Read the model definition and answer for the solid it produces. Units are mm, in the model's axes. Face numbers are marked on the shaded views. Coordinates: 2 decimals unless noted, no trailing zeros. Write each loop counter-clockwise with the first axis right and the second up, starting at its lowest first coordinate (ties: lowest second). Pieces come first, ordered by that corner, then holes. Notation, with made-up numbers: (4.5, -39.5) -> (56.5, -39.5) arc R11 ccw to (56.5, -31.5) -> close; hole circle Ø1 at (-16.5, 41.25). An arc over 180 degrees is marked (long way). Return JSON: item names as keys, results as strings.
from build123d import *

# Parameters (mm, degrees)
SKETCH1_R           = 6.1
SKETCH1_R_2         = 1.5
BOSS_EXTRUDE1_DEPTH = 2.3
SKETCH2_R           = 4.4
SKETCH2_R_2         = 3
BOSS_EXTRUDE2_DEPTH = 3.2
SKETCH3_R           = 0.75
BOSS_EXTRUDE3_DEPTH = 2.3
CIRPATTERN1_COUNT   = 6


with BuildPart() as part:
    # Sketch1 → Boss-Extrude1 (new body)
    with BuildSketch(Plane(origin=(0, 0, 0), x_dir=(1, 0, 0), z_dir=(0, 1, 0))):
        Circle(SKETCH1_R)
        Circle(SKETCH1_R_2, mode=Mode.SUBTRACT)
    extrude(amount=BOSS_EXTRUDE1_DEPTH)

    # Sketch2 → Boss-Extrude2 (add)
    with BuildSketch(Plane(origin=(0, 2.3, 0), x_dir=(1, 0, 0), z_dir=(0, 1, 0))):
        Circle(SKETCH2_R)
        Circle(SKETCH2_R_2, mode=Mode.SUBTRACT)
    extrude(amount=BOSS_EXTRUDE2_DEPTH)

    # Sketch3 → Boss-Extrude3 (add)
    with BuildSketch(Plane.XZ):
        with BuildLine():
            Line((-4.5, -4.118252056), (-2.468988638, -16.892549493))
            ThreePointArc((-2.468988638, -16.892549493), (0, -19), (2.468988638, -16.892549493))
            Line((2.468988638, -16.892549493), (4.5, -4.118252056))
            ThreePointArc((4.5, -4.118252056), (0, -6.1), (-4.5, -4.118252056))
        make_face()
        with Locations((0, -16)):
            Circle(SKETCH3_R, mode=Mode.SUBTRACT)
        with Locations((0, -13)):
            Circle(SKETCH3_R, mode=Mode.SUBTRACT)
        with Locations((0, -10)):
            Circle(SKETCH3_R, mode=Mode.SUBTRACT)
        with Locations((0, -7)):
            Circle(SKETCH3_R, mode=Mode.SUBTRACT)
    boss_extrude3 = extrude(amount=-BOSS_EXTRUDE3_DEPTH)

    # CirPattern1: Boss-Extrude3 ×6 about axis
    cirpattern1_axis = Axis((0, 0, 0), (0, 1, 0))
    for i in range(1, CIRPATTERN1_COUNT):
        add(boss_extrude3.rotate(cirpattern1_axis, i * 360 / CIRPATTERN1_COUNT))


solid = part.part
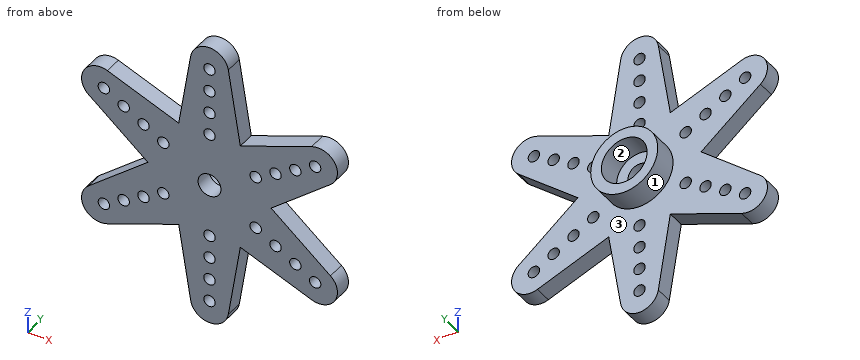
1. Consider L1, parallel to Y at x = 0.5, z = 6; L2, parallel to Z at x = -1, y = 3.65; L3, parallel to Z at x = 2.5, y = 4.1. Determine where each line is inside the solid, lowest interval first.
Taken from the geometry:
{"L1": "y = 0 to 2.3", "L2": "z = -4.28 to -2.83, 2.83 to 4.28", "L3": "z = -3.62 to -1.66, 1.66 to 3.62"}
2. The part is cut by section B-B (z = 16). Determine the outline of the cut face in (x, y), then the cut area to 3 significant figures.
Taken from the geometry:
{"outline": "(-2.61, 0) -> (-0.75, 0) -> (-0.75, 2.3) -> (-2.61, 2.3) -> close; (0.75, 0) -> (2.61, 0) -> (2.61, 2.3) -> (0.75, 2.3) -> close", "area": "8.56 mm2"}
3. The part is cut by section D-D (y = 1.8). Count the separate pieces of the cut face and the enclosed holes in it, then the cut area to 3 significant figures.
Taken from the geometry:
{"separate pieces": "1", "enclosed holes": "25", "area": "554 mm2"}
4. The part is cut by section A-A (z = 5). Determine the outline of the cut face in (x, y).
Taken from the geometry:
{"outline": "(-14.25, 0) -> (-9.41, 0) -> (-9.41, 2.3) -> (-14.25, 2.3) -> close; (-7.91, 0) -> (7.91, 0) -> (7.91, 2.3) -> (-7.91, 2.3) -> close; (9.41, 0) -> (14.25, 0) -> (14.25, 2.3) -> (9.41, 2.3) -> close"}
5. The part is cut by section C-C (y = 4.4). Determine the outline of the cut face in (x, z), then the cut area to 3 significant figures.
Taken from the geometry:
{"outline": "circle Ø8.8 at (0, 0); hole circle Ø6 at (0, 0)", "area": "32.5 mm2"}
6. For a pull along Z with two mould halves and no side action, classify the marked faces 1, 2 and 3 as +Z half, -Z half, draft (parallel to the pull), parting line (faces both ways), or undercut.
Taken from the geometry:
{"face 1": "parting line", "face 2": "undercut", "face 3": "draft"}
7. Flat-ended cylindrical pins translate along their axes: pin 1 Ø1.7 at (x, z) = (0, -7) entering from +Y; pin 2 Ø1.4 at (x, z) = (-8.66, 5) entering from -Y; pin 3 Ø2 at (y, z) = (3, 9.5) entering from +X. Find the tip coordinate at first contact, or state that the pin passes through.
Taken from the geometry:
{"pin 1": "stops at y = 2.3", "pin 2": "passes through", "pin 3": "stops at x = 16.73"}
